```python
from build123d import *

# Parameters (mm, degrees)
BOSS_EXTRUDE1_DEPTH = 45
SKETCH2_R           = 19.8
CUT_EXTRUDE1_DEPTH  = 42
CUT_EXTRUDE2_START  = -1.5
SKETCH3_R           = 19.8
CUT_EXTRUDE2_DEPTH  = 1.5
FILLET1_R           = 1
FILLET2_R           = 0.5
FILLET3_R           = 1
FILLET4_R           = 1
BOSS_EXTRUDE2_DEPTH = 1.5
FILLET5_R           = 0.2
FILLET6_R           = 0.5
FILLET7_R           = 0.5


with BuildPart() as part:
    # Sketch1 → Boss-Extrude1 (new body)
    with BuildSketch(Plane(origin=(0, 0, 0), x_dir=(1, 0, 0), z_dir=(0, 1, 0))):
        Polygon((8.732802634, -21.98002019), (21.717245289, -9.367197366), (21.98002019, 8.732802634), (9.367197366, 21.717245289), (-8.732802634, 21.98002019), (-21.717245289, 9.367197366), (-21.98002019, -8.732802634), (-9.367197366, -21.717245289), align=None)
    extrude(amount=BOSS_EXTRUDE1_DEPTH)

    # Sketch2 → Cut-Extrude1 (cut)
    with BuildSketch(Plane(origin=(0, 45, 0), x_dir=(1, 0, 0), z_dir=(0, 1, 0))):
        with Locations(Location((0, 0, 0), (0, 0, 270))):
            Circle(SKETCH2_R)
    extrude(amount=-CUT_EXTRUDE1_DEPTH, mode=Mode.SUBTRACT)

    # Sketch3 → Cut-Extrude2 (cut)
    with BuildSketch(Plane.XZ.offset(CUT_EXTRUDE2_START)):
        with Locations(Location((0, 0, 0), (0, 0, 90))):
            Circle(SKETCH3_R)
    extrude(amount=CUT_EXTRUDE2_DEPTH, mode=Mode.SUBTRACT)

    # Fillet1
    fillet1_edges = [part.edges().sort_by_distance(p)[0] for p in [
        (0, 0, -19.8),
    ]]
    fillet(fillet1_edges, radius=FILLET1_R)

    # Fillet2
    fillet2_edges = [part.edges().sort_by_distance(p)[0] for p in [
        (0, 1.5, -19.8),
    ]]
    fillet(fillet2_edges, radius=FILLET2_R - 0.0001)  # a hair under: the kernel refuses the full size

    # Fillet3
    fillet3_edges = [part.edges().sort_by_distance(p)[0] for p in [
        (21.848632739, 45, 0.317197366),
        (15.673608778, 45, -15.225023962),
        (0.317197366, 45, -21.848632739),
        (-15.225023962, 45, -15.673608778),
        (-21.848632739, 45, -0.317197366),
        (-15.673608778, 45, 15.225023962),
        (-0.317197366, 45, 21.848632739),
        (15.225023962, 45, 15.673608778),
    ]]
    fillet(fillet3_edges, radius=FILLET3_R)

    # Fillet4
    fillet4_edges = [part.edges().sort_by_distance(p)[0] for p in [
        (0, 45, -19.8),
    ]]
    fillet(fillet4_edges, radius=FILLET4_R)

    # Sketch4 → Boss-Extrude2 (add, symmetric)
    with BuildSketch(Plane.XY):
        with BuildLine():
            Line((21.717245289, 6.575350598), (33.933777265, 15.786558253))
            ThreePointArc((33.933777265, 15.786558253), (37.284614612, 31.928177441), (21.717245289, 37.353764349))
            ThreePointArc((21.717245289, 37.353764349), (21.300504514, 37.172559686), (20.8935235, 36.970385359))
            Line((20.8935235, 36.970385359), (21.490631851, 34.963416872))
            ThreePointArc((21.490631851, 34.963416872), (21.994919911, 35.192343489), (22.505339257, 35.407252623))
            ThreePointArc((22.505339257, 35.407252623), (35.457390534, 30.893164316), (32.669493861, 17.463337152))
            Line((32.669493861, 17.463337152), (20.452961885, 8.252129496))
            ThreePointArc((20.452961885, 8.252129496), (20.246714138, 6.781598345), (21.717245289, 6.575350598))
        make_face()
    extrude(amount=BOSS_EXTRUDE2_DEPTH, both=True)

    # Fillet5
    fillet5_edges = [part.edges().sort_by_distance(p)[0] for p in [
        (15.673608778, 0, -15.225023962),
        (21.848632739, 0, 0.317197366),
        (15.225023962, 0, 15.673608778),
        (-0.317197366, 0, 21.848632739),
        (-15.673608778, 0, 15.225023962),
        (-21.848632739, 0, -0.317197366),
        (-15.225023962, 0, -15.673608778),
        (0.317197366, 0, -21.848632739),
    ]]
    fillet(fillet5_edges, radius=FILLET5_R)

    # Fillet6
    fillet6_edges = [part.edges().sort_by_distance(p)[0] for p in [
        (27.882619067, 11.224013431, 1.5),
        (27.904395993, 11.24043313, -1.5),
        (37.31478879, 31.874600745, 1.5),
        (37.326195009, 31.854186297, -1.5),
    ]]
    fillet(fillet6_edges, radius=FILLET6_R)

    # Fillet7
    fillet7_edges = [part.edges().sort_by_distance(p)[0] for p in [
        (27.250477366, 13.3774242, 1.5),
        (35.457390534, 30.893164316, 1.5),
        (22.167087746, 35.266692743, 1.5),
    ]]
    fillet(fillet7_edges, radius=FILLET7_R)


solid = part.part
```
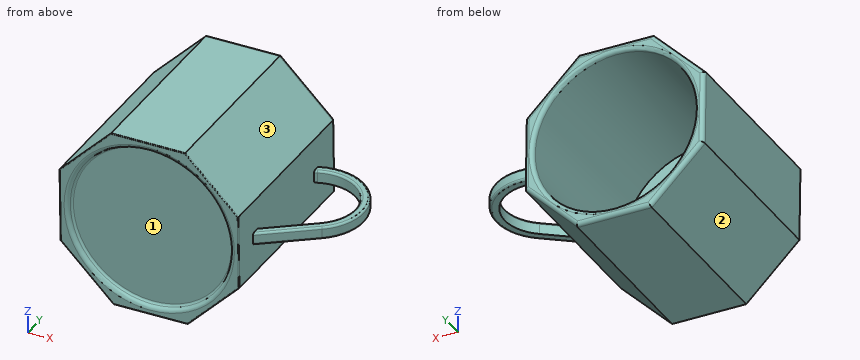
Design review of the part built by this model. Coordinates are the model's own, in mm. Face numbers are marked on the shaded views. Give positions to 0.01 mm unless a question says otherwise; leave off trailing zeros. Write each loop counter-clockwise with the first axis right and the second up, starting at its lowest first coordinate (ties: lowest second). Pieces come first, ordered by that corner, then holes.
(1) Wall thickness on line 1 along Y through (x, z) = (9, 7); line 2 along X through (y, z) = (14, 0); line 3 along X through (y, z) = (41, 3): over which ranges is each line inside the solid? List them lowest first.
Checked values:
line 1: y = 1.5 to 3
line 2: x = -21.85 to -19.8, 19.8 to 21.85, 28.08 to 31.56
line 3: x = -21.9 to -19.57, 19.57 to 21.81
(2) Clearance check with flat-ended pins moving along their axes: pin 1 Ø12 at (x, z) = (7.5, 15.5) entering from -Y; pin 2 Ø8 at (x, y) = (20, 20.5) entering from +Z; pin 3 Ø5 at (x, z) = (12, 4.5) entering from +Y; pin 4 Ø24 at (x, z) = (0, 0) entering from -Y. State where each tip first meets the part, or that it passes through.
Checked values:
pin 1: stops at y = 0
pin 2: stops at z = 14.92
pin 3: stops at y = 3
pin 4: stops at y = 1.5
(3) Mouldability with a two-part tool opening along X and no side actions: class the marked faces 1, 2 and 3 as +X half, -X half, draft (parallel to the pull), parting line (faces both ways), or undercut.
Checked values:
face 1: undercut
face 2: -X half
face 3: +X half
(4) Add section B-B (y = 23). Give the number of separate pieces and of enclosed holes in the cut face, and give its area (3 significant figures).
Checked values:
separate pieces: 2
enclosed holes: 1
area: 357 mm2
(5) Add section A-A (y = 39.5). Give the boundary of the cut face in (x, z).
Checked values:
outline: (-21.98, 8.73) - (-21.72, -9.37) - (-8.73, -21.98) - (9.37, -21.72) - (21.98, -8.73) - (21.72, 9.37) - (8.73, 21.98) - (-9.37, 21.72) - close; hole circle Ø39.6 at (0, 0)
